Autodesk Inventor part; units mm, degrees
ref_plane "YZ Plane" through (0, 0, 0) normal (1, 0, 0) x (0, 1, 0)
ref_plane "XZ Plane" through (0, 0, 0) normal (0, 1, 0) x (-1, 0, 0)
ref_plane "XY Plane" through (0, 0, 0) normal (0, 0, 1) x (1, 0, 0)
sketch "Sketch1" plane through (0, 0, 0) normal (0, 1, 0) x (-1, 0, 0)
  line L0 (10, -17.5) -> (-10, -17.5)
  line L1 (-10, -17.5) -> (-10, 18.5)
  line L2 (-10, 18.5) -> (10, 18.5)
  line L3 (10, 18.5) -> (10, -17.5)
  point P0 (0, 0)
  dimension "d0" = 20
  dimension "d1" = 36
  dimension "d2" = 17.5
  dimension "d3" = 10
extrude "Plate1" add sketch "Sketch1" along normal blind 1.5
sketch "Sketch2" plane through (-10, 0, -19) normal (0, 0, 1) x (1, 0, 0)
  line L0 (20, 0) -> (0, 0)
  line L1 (0, 0) -> (0, 46.6)
  line L2 (0, 46.6) -> (20, 46.6)
  line L3 (20, 46.6) -> (20, 0)
edge flange "Flange1" height 46.6 angle 90 thickness 1.5 bend radius 0.31 thickness toward (0, 0, 1) relief tear relief width 1.5 relief depth 0.75 edges at (0, 1.5, -17.5) wall of the first edge with corners at (10, 0, -19) (-10, 0, -19) (-10, 46.6, -19) (10, 46.6, -19)
bend "Bend1"
corner "Corner1"
sketch "Sketch3" plane through (10, 0, 20) normal (0, 0, -1) x (-1, 0, 0)
  line L0 (20, 0) -> (0, 0)
  line L1 (0, 0) -> (0, 46.6)
  line L2 (0, 46.6) -> (20, 46.6)
  line L3 (20, 46.6) -> (20, 0)
edge flange "Flange2" height 46.6 angle 90 thickness 1.5 bend radius 0.31 thickness toward (0, 0, -1) relief tear relief width 1.5 relief depth 0.75 edges at (0, 1.5, 18.5) wall of the first edge with corners at (-10, 0, 20) (10, 0, 20) (10, 46.6, 20) (-10, 46.6, 20)
bend "Bend2"
corner "Corner2"
sketch "Sketch4" plane through (-10, 46.6, 20) normal (0, 0, 1) x (1, 0, 0)
  circle A0 centre (10, -10) radius 10
  line L0 (0, 0) -> (20, 0)
  line L1 (0, 0) -> (20, 0)
  line L2 (20, 0) -> (20, -10)
  line L3 (20, -10) -> (0, -10)
  line L4 (0, -10) -> (0, 0)
  line L5 (0, -44.79) -> (0, 0)
  point P0 (10, -46.6)
  point P1 (10, -10)
  point P2 (20, 0)
  point P3 (10, 0)
  point P4 (0, -10)
  point P5 (8.5893, 0)
  point P6 (0, -10)
  dimension "d26" = 20
  dimension "d25" = 10
  dimension "d27" = 10
  dimension "d28" = 10
extrude "Extrusion1" cut sketch "Sketch4" against normal blind 10 contours L4 L0 A0 | A0 L0 L2
sketch "Sketch5" plane through (10, 46.6, -19) normal (0, 0, -1) x (-1, 0, 0)
  arc A0 (20, -10) -> (0, -10) centre (10, -10) ccw
  point P0 (10, -46.6)
hole "Hole1" at (0, 36.6, -19) direction (0, 0, 1) diameter 13.5 depth 1.5
sketch "Sketch6" plane through (10, 46.6, -19) normal (0, 0, -1) x (-1, 0, 0)
  circle A0 centre (10, -10) radius 6.75
  line L0 (0, 0) -> (20, 0)
  line L1 (0, -44.79) -> (0, 0)
  line L2 (24, 0) -> (-4, 0)
  line L3 (-4, 0) -> (-4, -9.9)
  line L4 (-4, -9.9) -> (24, -9.9)
  line L5 (24, -9.9) -> (24, 0)
  point P0 (10, -46.6)
  point P1 (20, 0)
  point P2 (6.005, 0)
  point P3 (13.995, 0)
  dimension "d38" = 9.9
  dimension "d39" = 4
  dimension "d40" = 28
extrude "Extrusion2" cut sketch "Sketch6" against normal blind 10 contours L4 A0 | A0 L4 L1 L0 L2 L5 | L4 L3 L2 L1 picked at (7.8223, -9.3675)
fillet "Fillet1" radius 1 2 edges at (-10, 36.7, -18.25) (10, 36.7, -18.25)
sketch "Sketch7" plane through (-10, 1.81, 20) normal (0, 0, 1) x (1, 0, 0)
  arc A0 (20, 34.79) -> (0, 34.79) centre (10, 34.79) ccw
  point P0 (10, -1.81)
hole "Hole2" at (0, 36.6, 20) direction (0, 0, -1) diameter 5.1 depth 1.5
sketch "Sketch8" plane through (0, 0, 0) normal (0, -1, 0) x (1, 0, 0)
  line L0 (2.55, 18.5) -> (-2.55, 18.5)
  line L1 (-10, 18.5) -> (10, 18.5)
  line L2 (10, 18.5) -> (-10, 18.5)
  line L3 (10, 18.19) -> (-10, 18.19)
  line L4 (-10, -17.19) -> (-10, 18.19)
  line L5 (-10, -17.19) -> (10, -17.19)
  line L6 (10, 18.19) -> (10, -17.19)
  point P0 (0, 0)
  point P1 (7, 9.5)
  point P2 (7, -4.5)
  point P3 (-7, 9.5)
  point P4 (-7, -4.5)
  dimension "d51" = 9
  dimension "d52" = 3
  dimension "d55" = 14
  dimension "d58" = 14
hole "Hole3" at (7, 0, 9.5) at (7, 0, -4.5) at (-7, 0, 9.5) at (-7, 0, -4.5) direction (0, 1, 0) diameter 3 depth 1.5
hole "Hole5" at (-8, 29.7, -17.5) at (8, 29.7, -17.5) at (7, 16.48, -17.5) at (-7, 16.48, -17.5) at (0, 9.18, -17.5) direction (0, 0, -1) diameter 2.1 depth 1.5
sketch "Sketch11" plane through (-10, 1.81, 20) normal (0, 0, 1) x (1, 0, 0)
  circle A0 centre (10, 7.37) radius 1.1
  point P0 (10, -1.81)
hole "Hole6" at (0, 9.18, 20) direction (0, 0, -1) diameter 3 depth 1.5
equation "\"d66\" = Thickness"
equation "\"d80\" = Thickness"
equation "\"d49\" = Thickness"
equation "\"d4\" = Thickness"
equation "\"d15\" = BendReliefWidth"
equation "\"d16\" = BendReliefDepth"
equation "\"d17\" = MinimumRemnant"
equation "\"d18\" = TransitionRadius"
equation "\"d21\" = BendRadius"
equation "\"d22\" = CornerReliefSize"
equation "\"d23\" = GapSize"
equation "\"d24\" = JacobiRadiusSize"
equation "\"d36\" = Thickness"
equation "\"d5\" = BendReliefWidth"
equation "\"d6\" = BendReliefDepth"
equation "\"d7\" = MinimumRemnant"
equation "\"d8\" = TransitionRadius"
equation "\"d11\" = BendRadius"
equation "\"d12\" = CornerReliefSize"
equation "\"d13\" = GapSize"
equation "\"d14\" = JacobiRadiusSize"
equation "\"d87\" = Thickness"
equation "\"BendReliefWidth\" = Thickness"
equation "\"BendReliefDepth\" = 0.5 * Thickness"
equation "\"CornerReliefSize\" = 4 * Thickness"
equation "\"MinimumRemnant\" = 2 * Thickness"
equation "\"TransitionRadius\" = BendRadius"
equation "\"JacobiRadiusSize\" = BendRadius"
equation "\"GapSize\" = Thickness"
properties part number "axis_9_bottom_frame" material "Aluminum 6061-AHC"
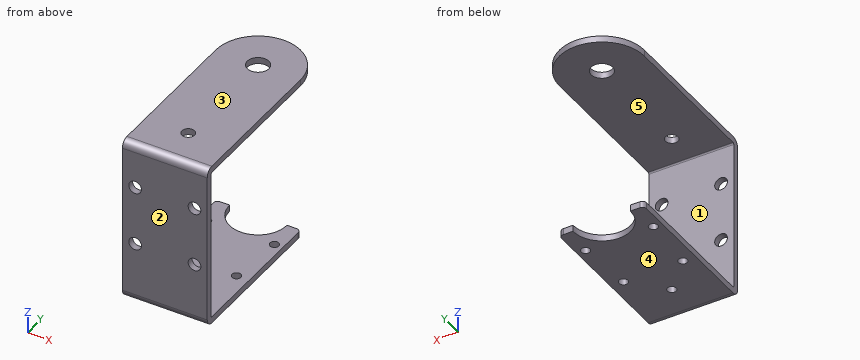
The listing builds one solid part. Answer for the finished solid, in the listing's coordinates (mm). Face numbers are marked on the shaded views. A direction names the side the tool comes from. Coordinates: 2 decimals unless noted, no trailing zeros. Loops run counter-clockwise (first coordinate to the right, second up) from the corner with the lowest first, then second, coordinate; pieces in that order, holes last. Notation, with made-up numbers: M -7.75,-33.5 L -3.75,-33.5 A31 ccw -3.75,5.5 Z; hole C -7.75,-26.5 d8. An arc over 180 degrees is marked long. Answer as CSV lines item,"result". Start each with the question number.
(1) For the marked faces 1 and 2, determine the directions among +Z, -Z, +X, -X, +Y, -Y from which every point of the face is accessible in a straight line to the end or side of a thin tool.
(2) The mould has two halves that part along Z. Classify the marked faces 3, 4 and 5: pulls with the +Z half, pulls with the -Z half, needs draft (parallel to the pull), parting line crosses it, or undercut.
(3) The part is cut by section C-C (x = 0). Give the vertices of the cut face in (y, z), and give its area (3 significant figures).
(4) Find the intervals of material crossed by L1, parallel to X at y = 0.7, z = 9.5; L2, parallel to Z at x = -6.5, y = 22.5; L3, parallel to X at y = 36.6, z = 18.95, in increasing order. Write a range as [from, to].
(5) Given pin 1 (1.8 mm diameter, centred on x = -7, z = -4.5, fed in from +Y); pin 2 (2.5 mm diameter, centred on x = 0, y = 9.18, fed in from +Z); pin 3 (0.8 mm diameter, centred on x = -8.5, z = -18.5, fed in from +Y); pin 4 (1.5 mm diameter, centred on x = -1, z = -10.5, fed in from +Y), each flat-ended and moving along its own axis, determine where each tip first touches the part or whether it passes through.
(6) The part is cut by section D-D (z = -7.5). Give the vertices of the cut face in (x, y), and give its area (3 significant figures).
(7) The part is cut by section B-B (y = 16.48). Give the vertices of the cut face in (x, z).
(8) The part is cut by section A-A (z = 9.5). Give the vertices of the cut face in (x, y).
Determined:
1,face 1,"+X, -X, +Y"
1,face 2,"+Z, -Z, +X, -X, -Y"
2,face 3,"pulls with the +Z half"
2,face 4,"pulls with the -Z half"
2,face 5,"undercut"
3,outline,"M 0,-17.19 A1.81 ccw 1.81,-19 L 8.13,-19 L 8.13,-17.5 L 1.81,-17.5 A0.31 cw 1.5,-17.19 L 1.5,18.19 A0.31 cw 1.81,18.5 L 7.68,18.5 L 7.68,20 L 1.81,20 A1.81 ccw 0,18.19 Z; M 10.23,-19 L 29.85,-19 L 29.85,-17.5 L 10.23,-17.5 Z; M 10.68,18.5 L 34.05,18.5 L 34.05,20 L 10.68,20 Z; M 39.15,18.5 L 46.6,18.5 L 46.6,20 L 39.15,20 Z"
3,area,"152 mm2"
4,L1,"[-10, -8.5], [-5.5, 5.5], [8.5, 10]"
4,L2,"[-19, -17.5], [18.5, 20]"
4,L3,"[-10, -2.55], [2.55, 10]"
5,pin 1,"through"
5,pin 2,"z = -17.5"
5,pin 3,"y = 36.7"
5,pin 4,"y = 1.5"
6,outline,"M -10,0 L 10,0 L 10,1.5 L -10,1.5 Z"
6,area,"30.0 mm2"
7,outline,"M -10,-19 L -8.05,-19 L -8.05,-17.5 L -10,-17.5 Z; M -10,18.5 L 10,18.5 L 10,20 L -10,20 Z; M -5.95,-19 L 5.95,-19 L 5.95,-17.5 L -5.95,-17.5 Z; M 8.05,-19 L 10,-19 L 10,-17.5 L 8.05,-17.5 Z"
8,outline,"M -10,0 L -8.5,0 L -8.5,1.5 L -10,1.5 Z; M -5.5,0 L 5.5,0 L 5.5,1.5 L -5.5,1.5 Z; M 8.5,0 L 10,0 L 10,1.5 L 8.5,1.5 Z"
